Can you work these out from the drawing? Everything is in mm from the part's minimum corner. A direction names the side the tool comes from. Coordinates: 2 decimals unless noted, no trailing zeros. Loops run counter-clockwise (first coordinate to the right, second up) from the corner with the lowest first, then second, coordinate; pieces in that order, holes last.
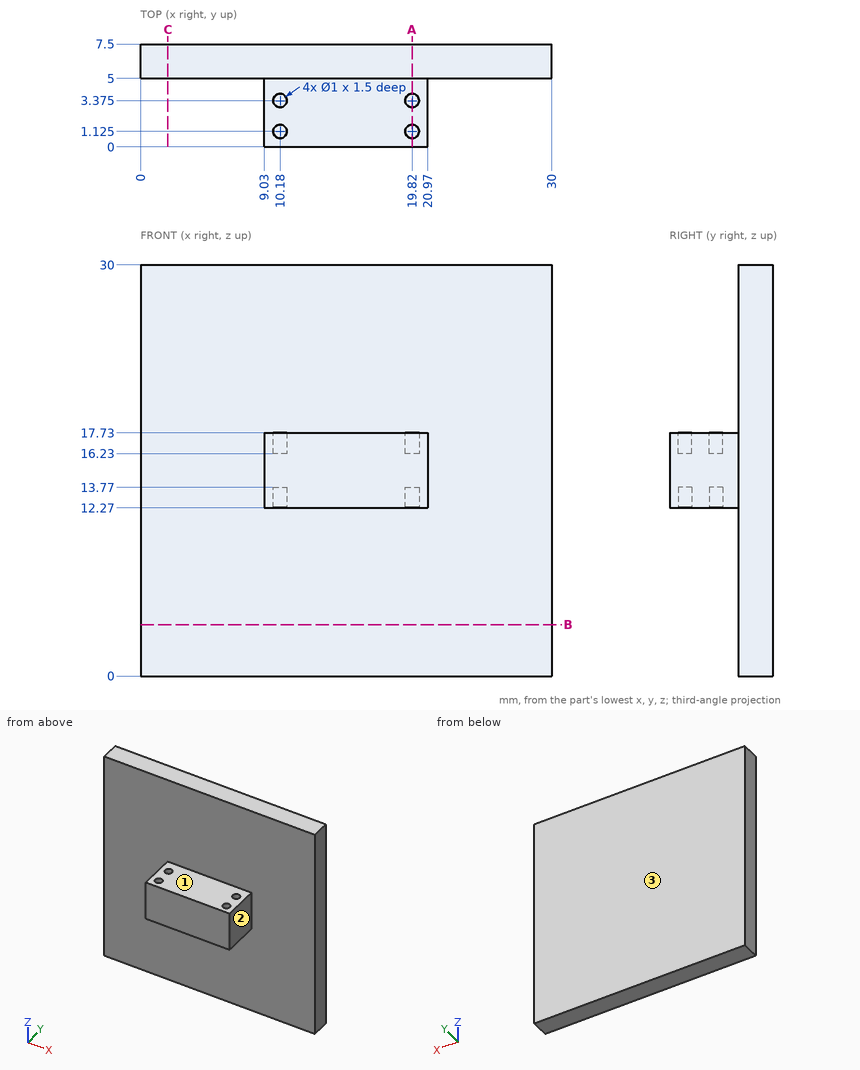
(1) Which directions (+Z, -Z, +X, -X, +Y, -Y) give clear straight access to the entire face, cutting with the end or side of a thin tool? Please do the marked faces 1, 2 and 3.
Answers:
face 1: +Z, +X, -X, -Y
face 2: +Z, -Z, +X, -Y
face 3: +Z, -Z, +X, -X, +Y
(2) Imagine slicing it at A-A, the plane x = 19.82. Write out the boundary of the cut face in (y, z) (3 decimals).
Answers:
outline: (0, 12.27) - (0.625, 12.27) - (0.625, 13.77) - (1.625, 13.77) - (1.625, 12.27) - (2.875, 12.27) - (2.875, 13.77) - (3.875, 13.77) - (3.875, 12.27) - (5, 12.27) - (5, 0) - (7.5, 0) - (7.5, 30) - (5, 30) - (5, 17.73) - (3.875, 17.73) - (3.875, 16.23) - (2.875, 16.23) - (2.875, 17.73) - (1.625, 17.73) - (1.625, 16.23) - (0.625, 16.23) - (0.625, 17.73) - (0, 17.73) - close
(3) I need wall thicknesses on probe 1 along Y at (x, z) = (19.82, 17.1) (3 decimals); probe 2 along Z at (x, y) = (17.5, 1.25); probe 3 along Y at (x, z) = (14.5, 7.5). Which ranges of each line are inside material? Lowest first, please.
Answers:
probe 1: y = 0 to 0.625, 1.625 to 2.875, 3.875 to 7.5
probe 2: z = 12.27 to 17.73
probe 3: y = 5 to 7.5
(4) Imagine slicing it at C-C, the plane x = 2. Write out the boundary of the cut face in (y, z), and give its area (3 significant figures).
Answers:
outline: (5, 0) - (7.5, 0) - (7.5, 30) - (5, 30) - close
area: 75.0 mm2
(5) For pin 1 (4 mm diameter, centred on x = 14, y = 3.5, fed in from -Z); pin 2 (2 mm diameter, centred on x = 21.5, z = 24, fed in from -Y); pin 3 (0.5 mm diameter, centred on x = 10, y = 3.5, fed in from -Z); pin 4 (1.5 mm diameter, centred on y = 2.5, z = 16, fed in from +X), each with a flat end and sliding along its axis, tell me the tip position at first contact or that it passes through.
Answers:
pin 1: stops at z = 0
pin 2: stops at y = 5
pin 3: stops at z = 13.77
pin 4: stops at x = 20.97
(6) Imagine slicing it at B-B, the plane z = 3.75. Write out the boundary of the cut face in (x, y).
Answers:
outline: (0, 5) - (30, 5) - (30, 7.5) - (0, 7.5) - close
